Geometry: final body of the model. Coordinates: model frame, mm. Face numbers are marked on the shaded views. A direction names the side the tool comes from. Give positions to 0.01 mm unless a question says otherwise; leave off trailing zeros. Write each loop counter-clockwise with the first axis right and the second up, starting at its lowest first coordinate (ties: lowest second). Pieces come first, ordered by that corner, then holes. Notation, with made-up numbers: (72, -34) - (98, -34) arc R18 ccw to (98, -15) - close; hole circle Ø2 at (61.25, 0.5). An arc over 180 degrees is marked (long way). Return JSON: item names as keys, results as strings.
Autodesk Inventor part; units mm, degrees
ref_plane "Work Plane1" through (0, 10, 39.5) normal (1, 0, 0) x (0, 0, -1)
ref_plane "YZ Plane" through (0, 0, 0) normal (1, 0, 0) x (0, 1, 0)
ref_plane "XZ Plane" through (0, 0, 0) normal (0, 1, 0) x (-1, 0, 0)
sketch "Sketch1" plane through (0, 0, 0) normal (0, 1, 0) x (-1, 0, 0)
  line L0 (15, 30) -> (-15, 30)
  line L1 (-15, 30) -> (-15, -30)
  line L2 (-15, -30) -> (15, -30)
  line L3 (15, -30) -> (15, 30)
  line L4 (15, 30) -> (-15, -30) construction
  line L5 (-15, 30) -> (15, -30) construction
  circle A0 centre (15, 30) radius 1.5
  circle A1 centre (15, 0) radius 1.5
  circle A2 centre (15, -30) radius 1.5
  circle A3 centre (-15, -30) radius 1.5
  circle A4 centre (-15, 0) radius 1.5
  circle A5 centre (-15, 30) radius 1.5
  line L6 (22.5, 39.5) -> (-22.5, 39.5)
  line L7 (-22.5, 39.5) -> (-22.5, -39.5)
  line L8 (-22.5, -39.5) -> (22.5, -39.5)
  line L9 (22.5, -39.5) -> (22.5, 39.5)
  line L10 (22.5, 39.5) -> (-22.5, -39.5) construction
  line L11 (-22.5, 39.5) -> (22.5, -39.5) construction
  point P0 (0, 0)
  dimension "d0" = 30
  dimension "d1" = 60
  dimension "d2" = 3
  dimension "d3" = 3
  dimension "d4" = 3
  dimension "d5" = 3
  dimension "d6" = 3
  dimension "d7" = 3
  dimension "d8" = 7.5
  dimension "d9" = 9.5
sketch "Sketch1 outline for Extrusion1" plane through (0, 0, 0) normal (0, 1, 0) x (-1, 0, 0)
  line L0 (22.5, 39.5) -> (-22.5, 39.5)
  line L1 (22.5, -39.5) -> (22.5, 39.5)
  line L2 (-22.5, 39.5) -> (-22.5, -39.5)
  line L3 (-22.5, -39.5) -> (22.5, -39.5)
  circle A0 centre (-15, -30) radius 1.5
  circle A1 centre (15, -30) radius 1.5
  circle A2 centre (-15, 0) radius 1.5
  circle A3 centre (-15, 30) radius 1.5
  circle A4 centre (15, 0) radius 1.5
  circle A5 centre (15, 30) radius 1.5
extrude "Extrusion1" add sketch "Sketch1 outline for Extrusion1" along normal blind 10
chamfer "Chamfer1" distance 2 angle 45 6 edges at (-13.5, 10, 30) (-13.5, 10, 0) (-13.5, 10, -30) (16.5, 10, -30) (16.5, 10, 0) (16.5, 10, 30)
sketch "Sketch2" plane through (0, 0, 0) normal (0, -1, 0) x (1, 0, 0)
  line L0 (-22.5, 39.5) -> (22.5, 39.5)
  line L1 (22.5, 39.5) -> (28.5, 39.5)
  line L2 (28.5, 39.5) -> (28.5, -39.5)
  line L3 (28.5, -39.5) -> (22.5, -39.5)
  line L4 (22.5, -39.5) -> (22.5, 39.5)
  line L5 (-22.5, -39.5) -> (-22.5, 39.5)
  line L6 (-22.5, 39.5) -> (-35, 39.5)
  line L7 (-35, 39.5) -> (-35, -39.5)
  line L8 (-35, -39.5) -> (-22.5, -39.5)
  line L9 (-22.5, -39.5) -> (-22.5, 39.5)
  line L10 (22.5, -39.5) -> (-22.5, -39.5)
  line L11 (-7.5, 39.5) -> (7.5, 39.5)
  line L12 (7.5, 39.5) -> (7.5, -39.5)
  line L13 (7.5, -39.5) -> (-7.5, -39.5)
  line L14 (-7.5, -39.5) -> (-7.5, 39.5)
  point P0 (0, 0)
  point P1 (7.5, 39.5)
  dimension "d15" = 6
  dimension "d16" = 12.5
  dimension "d19" = 15
  dimension "d20" = 15
sketch "Sketch2 outline for Extrusion2" plane through (0, 0, 0) normal (0, -1, 0) x (1, 0, 0)
  line L0 (-7.5, 39.5) -> (-7.5, -39.5)
  line L1 (7.5, 39.5) -> (-7.5, 39.5)
  line L2 (7.5, -39.5) -> (7.5, 39.5)
  line L3 (-7.5, -39.5) -> (7.5, -39.5)
  line L4 (-22.5, 39.5) -> (-35, 39.5)
  line L5 (-22.5, -39.5) -> (-22.5, 39.5)
  line L6 (-35, -39.5) -> (-22.5, -39.5)
  line L7 (-35, 39.5) -> (-35, -39.5)
  line L8 (22.5, 39.5) -> (22.5, -39.5)
  line L9 (28.5, 39.5) -> (22.5, 39.5)
  line L10 (28.5, -39.5) -> (28.5, 39.5)
  line L11 (22.5, -39.5) -> (28.5, -39.5)
extrude "Extrusion2" add sketch "Sketch2 outline for Extrusion2" against normal blind 40
sketch "Sketch3" plane through (28.5, 0, 39.5) normal (1, 0, 0) x (0, 0, -1)
  line L0 (0, 40) -> (79, 40)
  line L1 (39.5, 40) -> (39.5, 27.5)
  circle A0 centre (39.5, 27.5) radius 8.125
  circle A1 centre (39.5, 27.5) radius 3
  point P0 (39.5, 0)
  dimension "d21" = 16.25
  dimension "d22" = 12.5
  dimension "d23" = 6
sketch "Sketch3 outline for Extrusion3" plane through (28.5, 0, 39.5) normal (1, 0, 0) x (0, 0, -1)
  circle A0 centre (39.5, 27.5) radius 3
extrude "Extrusion3" cut sketch "Sketch3 outline for Extrusion3" against normal blind 110.5
chamfer "Chamfer2" distance 20 angle 45 6 edges at (25.5, 40, -39.5) (0, 40, -39.5) (-28.75, 40, -39.5) (-28.75, 40, 39.5) (0, 40, 39.5) (25.5, 40, 39.5)
sketch "Sketch4" plane through (-35, 10, -39.5) normal (-1, 0, 0) x (0, 0, 1)
  circle A0 centre (39.5, 17.5) radius 3
  circle A1 centre (39.5, 17.5) radius 4.15
  line L0 (37.435418, 13.9) -> (41.564582, 13.9)
  point P0 (39.5, -10)
  dimension "d29" = 8.3
  dimension "d63" = 3.6
sketch "Sketch4 outline for Extrusion4" plane through (-35, 10, -39.5) normal (-1, 0, 0) x (0, 0, 1)
  line L0 (37.435418, 13.9) -> (41.564582, 13.9)
  arc A0 (41.564582, 13.9) -> (37.435418, 13.9) centre (39.5, 17.5) ccw
  circle A1 centre (39.5, 17.5) radius 3
extrude "Extrusion4" cut sketch "Sketch4 outline for Extrusion4" against normal blind 15
sketch "Sketch5" plane through (-35, 10, -39.5) normal (-1, 0, 0) x (0, 0, 1)
  line L0 (35.875, 7) -> (43.125, 7)
  line L1 (43.125, 7) -> (43.125, 3.5)
  line L2 (43.125, 3.5) -> (35.875, 3.5)
  line L3 (35.875, 3.5) -> (35.875, 7)
  circle A0 centre (39.5, 17.5) radius 3
  line L4 (20, 30) -> (59, 30)
  point P0 (39.5, -10)
  dimension "d33" = 7.25
  dimension "d34" = 3.5
  dimension "d35" = 3.625
  dimension "d36" = 23
sketch "Sketch5 outline for Extrusion5" plane through (-35, 10, -39.5) normal (-1, 0, 0) x (0, 0, 1)
  line L0 (35.875, 7) -> (35.875, 3.5)
  line L1 (43.125, 7) -> (35.875, 7)
  line L2 (43.125, 3.5) -> (43.125, 7)
  line L3 (35.875, 3.5) -> (43.125, 3.5)
extrude "Extrusion5" cut sketch "Sketch5 outline for Extrusion5" against normal blind 15
sketch "Sketch6" plane through (0, 0, 0) normal (0, 1, 0) x (1, 0, 0)
  circle A0 centre (-28.75, 0) radius 2
  line L0 (-35, 19.5) -> (-35, -19.5)
  point P0 (0, 0)
  dimension "d42" = 4
  dimension "d43" = 6.25
sketch "Sketch6 outline for Extrusion6" plane through (0, 0, 0) normal (0, 1, 0) x (1, 0, 0)
  circle A0 centre (-28.75, 0) radius 2
extrude "Extrusion6" cut sketch "Sketch6 outline for Extrusion6" along normal blind 26.5
sketch "Sketch4 outline for Extrusion7" plane through (-35, 10, -39.5) normal (-1, 0, 0) x (0, 0, 1)
  circle A0 centre (39.5, 17.5) radius 4.15
extrude "Extrusion7" cut sketch "Sketch4 outline for Extrusion7" against normal blind 2
sketch "Sketch7" plane through (-35, 0, -39.5) normal (-1, 0, 0) x (0, 0, 1)
  circle A0 centre (39.5, 27.5) radius 3
  circle A1 centre (39.5, 27.5) radius 10.5
  circle A2 centre (39.5, 27.5) radius 17.5
  point P0 (39.5, 0)
  dimension "d46" = 21
  dimension "d47" = 35
sketch "Sketch7 outline for Extrusion8" plane through (-35, 0, -39.5) normal (-1, 0, 0) x (0, 0, 1)
  circle A0 centre (39.5, 27.5) radius 17.5
  circle A1 centre (39.5, 27.5) radius 10.5
extrude "Extrusion8" cut sketch "Sketch7 outline for Extrusion8" against normal blind 1.5
sketch "Sketch8" plane through (7.5, 10, 39.5) normal (1, 0, 0) x (0, 0, -1)
  circle A0 centre (39.5, 17.5) radius 3
  circle A1 centre (39.5, 17.5) radius 8.125
  point P0 (39.5, -10)
  dimension "d50" = 16.25
sketch "Sketch8 outline for Extrusion9" plane through (7.5, 10, 39.5) normal (1, 0, 0) x (0, 0, -1)
  circle A0 centre (39.5, 17.5) radius 8.125
  circle A1 centre (39.5, 17.5) radius 3
extrude "Extrusion9" cut sketch "Sketch8 outline for Extrusion9" against normal blind 5
ref_plane "Work Plane1" through (0, 10, 39.5) normal (1, 0, 0) x (0, 0, -1)
sketch "Sketch9" plane through (28.5, 0, 39.5) normal (1, 0, 0) x (0, 0, -1)
  circle A0 centre (26.094222, 16.251217) radius 4.5
  circle A1 centre (26.094222, 16.251217) radius 1.5
  circle A2 centre (39.5, 27.5) radius 3
  line L0 (39.5, 27.5) -> (11.266144, 27.5)
  arc A3 (41.564582, 23.9) -> (37.435418, 23.9) centre (39.5, 27.5) ccw
  line L1 (39.5, 27.5) -> (26.094222, 16.251217)
  point P0 (39.5, 0)
  dimension "d53" = 9
  dimension "d54" = 3
  dimension "d55" = 17.5
  dimension "d60" = 40
sketch "Sketch9 outline for Extrusion10" plane through (28.5, 0, 39.5) normal (1, 0, 0) x (0, 0, -1)
  circle A0 centre (26.094222, 16.251217) radius 1.5
extrude "Extrusion10" cut sketch "Sketch9 outline for Extrusion10" against normal blind 10
sketch "Sketch9 outline for Extrusion11" plane through (28.5, 0, 39.5) normal (1, 0, 0) x (0, 0, -1)
  circle A0 centre (26.094222, 16.251217) radius 4.5
  circle A1 centre (26.094222, 16.251217) radius 1.5
extrude "Extrusion11" cut sketch "Sketch9 outline for Extrusion11" against normal blind 3.5
sketch "Sketch10" plane through (0, 40, 0) normal (0, 1, 0) x (1, 0, 0)
  line L0 (-33.5, -12.247449) -> (-35, -12.247449)
  line L1 (-35, -12.247449) -> (-35, -19.5)
  line L2 (-22.5, -19.5) -> (-35, -19.5)
  line L3 (-22.5, -19.5) -> (-22.5, 19.5)
  line L4 (-35, 19.5) -> (-22.5, 19.5)
  line L5 (-35, 19.5) -> (-35, 12.247449)
  line L6 (-35, 12.247449) -> (-33.5, 12.247449)
  line L7 (-33.5, 12.247449) -> (-33.5, -12.247449)
  line L8 (-22.5, 39.5) -> (-22.5, -39.5)
  line L9 (-35, 12.247449) -> (-22.5, 12.247449)
  line L10 (-22.5, 12.247449) -> (-22.5, -12.247449)
  line L11 (-22.5, -12.247449) -> (-35, -12.247449)
  line L12 (-35, -12.247449) -> (-35, 12.247449)
  point P0 (0, 0)
sketch "Sketch10 outline for Extrusion12" plane through (0, 40, 0) normal (0, 1, 0) x (1, 0, 0)
  line L0 (-33.5, -12.247449) -> (-22.5, -12.247449)
  line L1 (-33.5, 12.247449) -> (-33.5, -12.247449)
  line L2 (-22.5, 12.247449) -> (-33.5, 12.247449)
  line L3 (-22.5, -12.247449) -> (-22.5, 12.247449)
extrude "Extrusion12" add sketch "Sketch10 outline for Extrusion12" along normal blind 3
fillet "Fillet1" radius 5 2 edges at (-28, 40, -12.2474) (-28, 40, 12.2474)
properties part number "Gimbal_2"
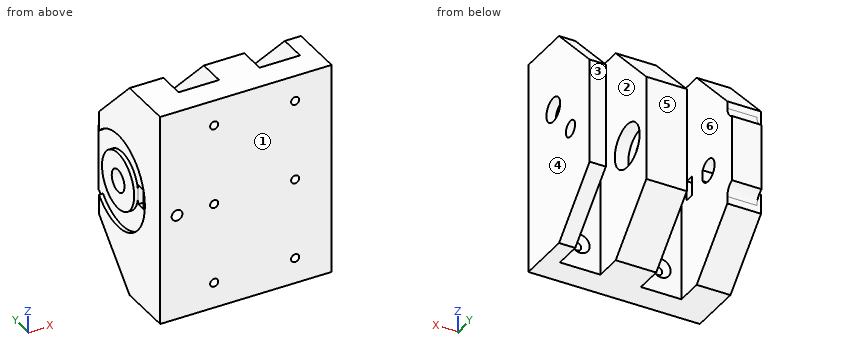
Q1. Pin query (flat end, axial travel): P1, Ø4.5, axis at y = 17, z = 13.5, coming from the +X side; P2, Ø2.5, axis at x = -28.75, z = 0, coming from the -Y side; P3, Ø5, axis at x = -3, y = 35.5, coming from the -Z side; P4, Ø24, axis at y = 28, z = -1.5, coming from the +X side. Return the tip coordinate at first contact, or that it passes through.
Answer key:
{"P1": "stops at x = 25", "P2": "stops at y = 31.46", "P3": "stops at z = -26.5", "P4": "stops at x = 28.5"}
Q2. Section query B-B, the plane x = 15. Return the cut outline in (y, z).
Answer key:
{"outline": "(0, -39.5) - (10, -39.5) - (10, -33.5) - (8, -31.5) - (0, -31.5) - close; (0, -28.5) - (8, -28.5) - (10, -26.5) - (10, -3.5) - (8, -1.5) - (0, -1.5) - close; (0, 1.5) - (8, 1.5) - (10, 3.5) - (10, 26.5) - (8, 28.5) - (0, 28.5) - close; (0, 31.5) - (8, 31.5) - (10, 33.5) - (10, 39.5) - (0, 39.5) - close"}
Q3. Mould query, pull axis X, two halves, no side actions, for the marked faces 4, 5 and 6. Classes: pulls with the +X half, pulls with the -X half, needs draft (parallel to the pull), parting line crosses it, or undercut.
Answer key:
{"face 4": "pulls with the +X half", "face 5": "needs draft", "face 6": "undercut"}
Q4. Material intervals for probe 1 along X at (y, z) = (37.5, -5.5); probe 2 along X at (y, z) = (33.5, -18); probe 3 along Y at (x, z) = (-1.75, 0), sorted ascending. Write a range as [from, to].
Answer key:
{"probe 1": "x = [-33.5, -22.5], [-7.5, 7.5], [22.5, 28.5]", "probe 2": "x = [-35, -22.5], [-7.5, 7.5], [22.5, 28.5]", "probe 3": "y = [0, 24.5], [30.5, 40]"}
Q5. Section query C-C, the plane x = -28.75. Return the cut outline in (y, z) (3 decimals).
Answer key:
{"outline": "(0, -39.5) - (20, -39.5) - (40, -19.5) - (40, -16.83) arc R5 cw to (43, -12.247) - (43, 12.247) arc R5 cw to (40, 16.83) - (40, 19.5) - (20, 39.5) - (0, 39.5) - (0, 2) - (13.5, 2) - (13.5, 3.625) - (17, 3.625) - (17, 2) - (23.9, 2) - (23.9, 2.065) arc R4.15 cw (long way) to (23.9, -2.065) - (23.9, -2) - (17, -2) - (17, -3.625) - (13.5, -3.625) - (13.5, -2) - (0, -2) - close"}
Q6. Set-up query: the marked faces 1, 2 and 3. Return all of +Z, -Z, +X, -X, +Y, -Y with unobstructed straight access to the full face (end or side cutting, diameter ignored); none if empty.
Answer key:
{"face 1": "+Z, -Z, +X, -X, -Y", "face 2": "+Z, -Z, +Y", "face 3": "+Z, -Z, +X, +Y"}
Q7. Section query D-D, the plane z = 20.5. Return the cut outline in (x, y), plus the area to 3 significant figures.
Answer key:
{"outline": "(-35, 0) - (28.5, 0) - (28.5, 39) - (22.5, 39) - (22.5, 10) - (7.5, 10) - (7.5, 39) - (-7.5, 39) - (-7.5, 10) - (-22.5, 10) - (-22.5, 39) - (-35, 39) - close", "area": "1,610 mm^2"}
Q8. Section query A-A, the plane z = 30. Return the cut outline in (x, y).
Answer key:
{"outline": "(-35, 0) - (-16.5, 0) - (-16.5, 8) - (-18.5, 10) - (-22.5, 10) - (-22.5, 29.5) - (-35, 29.5) - close; (-13.5, 0) - (13.5, 0) - (13.5, 8) - (11.5, 10) - (7.5, 10) - (7.5, 29.5) - (-7.5, 29.5) - (-7.5, 10) - (-11.5, 10) - (-13.5, 8) - close; (16.5, 0) - (28.5, 0) - (28.5, 29.5) - (22.5, 29.5) - (22.5, 10) - (18.5, 10) - (16.5, 8) - close"}
